The model under review builds one solid part; all positions refer to its coordinate system, in mm. Face numbers are marked on the shaded views. A direction names the side the tool comes from. Round coordinates to 2 decimals unless told otherwise and drop trailing zeros. Write each loop counter-clockwise with the first axis right and the second up, starting at its lowest first coordinate (ties: lowest second). Pieces come first, ordered by that corner, then holes. Notation, with made-up numbers: (-35, 60) - (-17, 60) arc R25 ccw to (-17, 97) - close; hole circle Ø6 at (-31, 9.25). An arc over 180 degrees is marked (long way). Use one line per item in the form item = value.
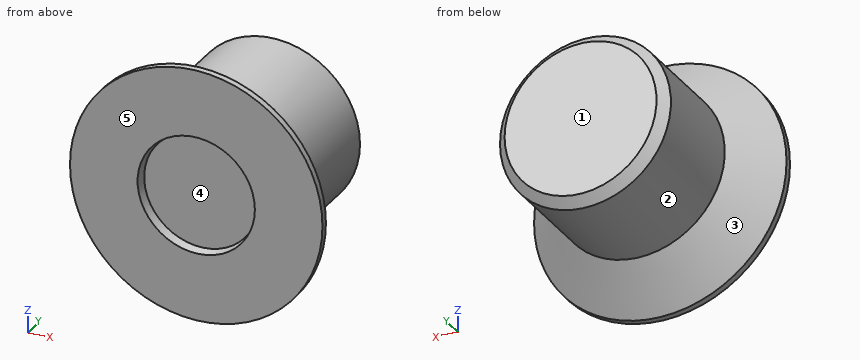
from build123d import *

# Parameters (mm, degrees)
CHAMFER1_SIZE  = 0.25
CHAMFER2_SIZE  = 0.25
CHAMFER2_SIZE2 = 0.176776695


with BuildPart() as part:
    # Sketch1 → Revolve1 (revolve)
    with BuildSketch(Plane.XY):
        Polygon((0, 0.25), (1.5, 0.25), (1.544081745, 0), (3.5, 0), (2.25, 1.25), (2.25, 4.25), (0, 4.25), align=None)
    revolve(axis=Axis((0, -277.798061763, 0), (0, 1, 0)))

    # Chamfer1
    chamfer1_edges = [part.edges().sort_by_distance(p)[0] for p in [
        (-2.25, 4.25, 0),
    ]]
    chamfer(chamfer1_edges, length=CHAMFER1_SIZE)

    # Chamfer2
    chamfer2_edges = [part.edges().sort_by_distance(p)[0] for p in [
        (-3.5, 0, 0),
    ]]
    chamfer2_side = [part.faces().sort_by_distance(p)[0] for p in [
        (-2.875, 0.625, 0),
    ]]
    chamfer(chamfer2_edges, length=CHAMFER2_SIZE, length2=CHAMFER2_SIZE2, reference=chamfer2_side[0])


solid = part.part
(1) The part is to be moulded in two halves that separate along Z. For the marked faces 3, 4 and 5, say which applies: +Z half, -Z half, draft (parallel to the pull), parting line (faces both ways), or undercut.
Geometry results:
face_3 = parting line
face_4 = undercut
face_5 = draft
(2) Machinability: for the marked faces 1 and 2, which of the approach directions +Z, -Z, +X, -X, +Y, -Y give a long, thin tool a straight path to every point of the face, cutting with its end or side? Answer none if there is none.
Geometry results:
face_1 = +Z, -Z, +X, -X, +Y
face_2 = +Y
(3) Insertion check: P1, Ø1.5, axis at y = 1, z = 0.5, coming from the -X side; P2, Ø1.5, axis at x = 1, y = 1, coming from the +Z side; P3, Ø1.5, axis at x = -2.5, y = 3, coming from the -Z side. Each pin has a flat end and moves straight along its axis. Give the tip position at first contact, or say it passes through.
Geometry results:
P1 = -3.22
P2 = 3.12
P3 = -1.41
(4) To check wall thickness, follow L1, parallel to Y at x = -1, z = -0.5; L2, parallel to Y at x = 1.25, z = 3; L3, parallel to Z at x = 0, y = 2.25. State the ranges of each line that lie inside material, in increasing order.
Geometry results:
L1 = 0.25 to 4.25
L2 = 0 to 0.25
L3 = -2.25 to 2.25
(5) Add section A-A on y = 2.65. Write out the cut boundary in (x, z).
Geometry results:
outline = circle Ø4.5 at (0, 0)
